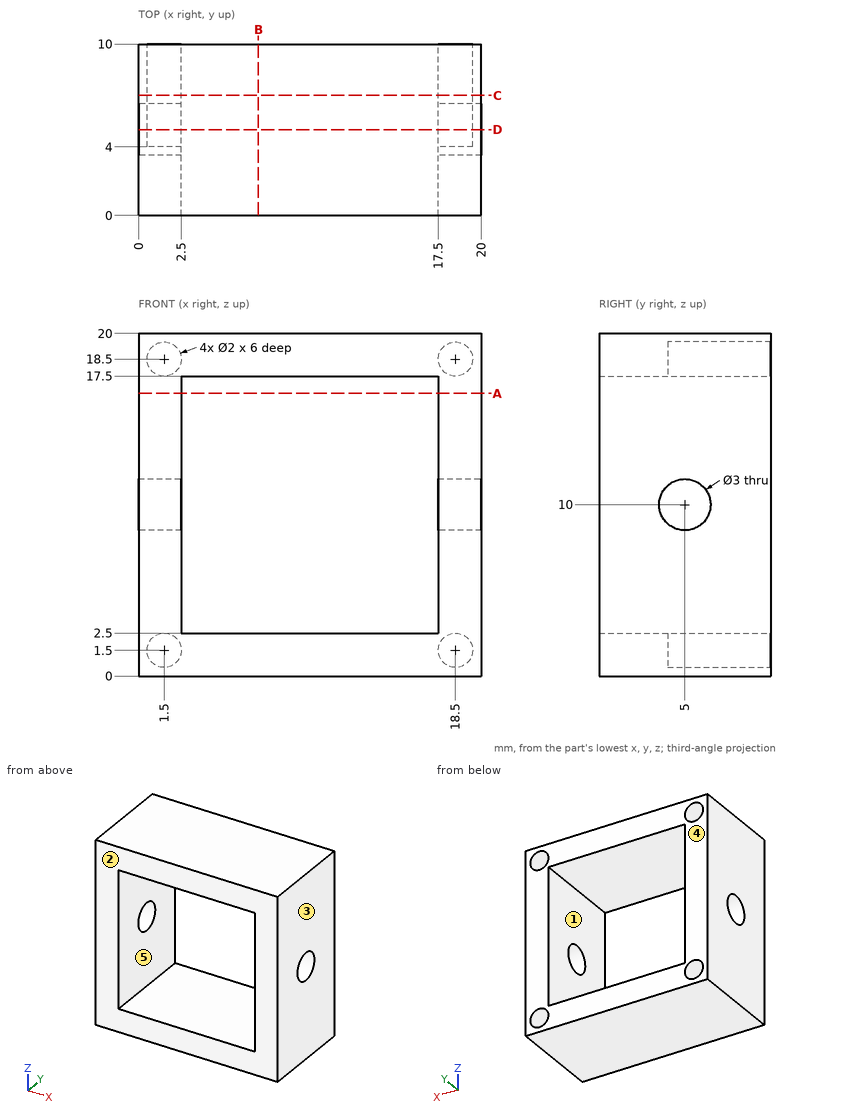
Can you work these out from the drawing? Everything is in mm from the part's minimum corner. A direction names the side the tool comes from. Give positions to 0.01 mm unless a question says otherwise; leave off trailing zeros. Write each loop counter-clockwise with the first axis right and the second up, starting at its lowest first coordinate (ties: lowest second). Pieces come first, ordered by that corner, then holes. Notation, with made-up numbers: M 6,18.25 L 51,18.25 A28 cw 51,57.25 Z; hole C -35,2.25 d6. An arc over 180 degrees is marked long. Answer in a Markdown table with one row per item. Add a question column.
Item 1: We'd pull the mould along X, two halves only. Please class the marked faces 3, 4 and 5: released by +X, released by -X, zero draft, split by the parting line, or undercut.
Item 2: Imagine slicing it at C-C, the plane y = 7. Write out the boundary of the cut face in (x, z), plus the area to 3 significant figures.
Item 3: For pin 1 Ø1.6 at (x, z) = (1.5, 1.5) entering from +Y; pin 2 Ø1.8 at (y, z) = (5, 10) entering from +X, each with a flat end and sliding along its axis, tell me the tip position at first contact or that it passes through.
Item 4: On a 3-axis mill with a long thin cutter (end or side, diameter ignored), from which of +Z, -Z, +X, -X, +Y, -Y can I reach the whole of each face in a straight line? I mean the marked faces 1 and 2. Say none if no direction works.
Item 5: Imagine slicing it at D-D, the plane y = 5. Write out the boundary of the cut face in (x, z).
Item 6: Imagine slicing it at A-A, the plane z = 16.5. Write out the boundary of the cut face in (x, y), plus the area to 3 significant figures.
Item 7: Imagine slicing it at B-B, the plane x = 7. Write out the boundary of the cut face in (y, z), plus the area to 3 significant figures.
Item 8: Please list where these lines run through material, in increasing order: L1, parallel to X at y = 2, z = 15; L2, parallel to Y at x = 18.85, z = 10.
Evaluation:
| question | item | result |
|---|---|---|
| 1 | face 3 | released by +X |
| 1 | face 4 | zero draft |
| 1 | face 5 | undercut |
| 2 | outline | M 0,0 L 20,0 L 20,20 L 0,20 Z; hole C 1.5,1.5 d2; hole C 1.5,18.5 d2; hole M 2.5,2.5 L 17.5,2.5 L 17.5,17.5 L 2.5,17.5 Z; hole C 18.5,1.5 d2; hole C 18.5,18.5 d2 |
| 2 | area | 162 mm² |
| 3 | pin 1 | stops at y = 4 |
| 3 | pin 2 | passes through |
| 4 | face 1 | +Y, -Y |
| 4 | face 2 | +Z, -Z, +X, -X, -Y |
| 5 | outline | M 0,0 L 20,0 L 20,8.5 L 17.5,8.5 L 17.5,2.5 L 2.5,2.5 L 2.5,8.5 L 0,8.5 Z; M 0,11.5 L 2.5,11.5 L 2.5,17.5 L 17.5,17.5 L 17.5,11.5 L 20,11.5 L 20,20 L 0,20 Z; hole C 1.5,1.5 d2; hole C 1.5,18.5 d2; hole C 18.5,1.5 d2; hole C 18.5,18.5 d2 |
| 6 | outline | M 0,0 L 2.5,0 L 2.5,10 L 0,10 Z; M 17.5,0 L 20,0 L 20,10 L 17.5,10 Z |
| 6 | area | 50.0 mm² |
| 7 | outline | M 0,0 L 10,0 L 10,2.5 L 0,2.5 Z; M 0,17.5 L 10,17.5 L 10,20 L 0,20 Z |
| 7 | area | 50.0 mm² |
| 8 | L1 | x = 0 to 2.5, 17.5 to 20 |
| 8 | L2 | y = 0 to 3.5, 6.5 to 10 |
